Geometry: final body of the model. Coordinates: model frame, mm. Face numbers are marked on the shaded views. A direction names the side the tool comes from. Give positions to 0.01 mm unless a question says otherwise; leave off trailing zeros. Loops run counter-clockwise (first coordinate to the right, second up) from the corner with the lowest first, then second, coordinate; pieces in that order, holes last.
1. First-contact query: P1, Ø8, axis at y = 19.5, z = 1, coming from the +X side; P2, Ø6, axis at y = 23.5, z = 1, coming from the -X side. Flat tips, straight axial feed; report the tip coordinate or a pass-through.
2. Material intervals for line 1 along Y through (x, z) = (-0.75, 6.25); line 2 along Z through (x, y) = (-1.75, 23.5); line 3 along Y through (x, z) = (-2, -3), sorted ascending.
3. Section B-B, the plane y = 22. Output: boundary loops of the cut face in (x, z), then the cut area to 3 significant figures.
4. Section A-A, the plane y = 31. Output: boundary loops of the cut face in (x, z).
5. Access query for the marked faces 1 and 2. Directions: +Z, -Z, +X, -X, +Y, -Y. A direction counts if a zero-diameter tool reaches every point of the face in a straight line with its end or side. Return the directions, or none.
from build123d import *

# Parameters (mm, degrees)
SKETCH1_W           = 4
SKETCH1_H           = 30
BOSS_EXTRUDE1_DEPTH = 5.5
FILLET1_R           = 0.4
CHAMFER1_SIZE       = 0.4
SKETCH3_OUTSIDE_W   = 25.696
SKETCH3_OUTSIDE_H   = 27.708
SKETCH3_OUTSIDE_R   = 6.5
CUT_EXTRUDE1_DEPTH  = 1
CUT_EXTRUDE1_DRAFT  = -52


with BuildPart() as part:
    # Sketch1 → Revolve1 (revolve)
    with BuildSketch(Plane.XY, mode=Mode.PRIVATE) as revolve1_sk:
        with Locations((-2, 15)):
            Rectangle(SKETCH1_W, SKETCH1_H)
    revolve(revolve1_sk.sketch.rotate(Axis((0, 30, 0), (0, -1, 0)), 270), axis=Axis((0, 30, 0), (0, -1, 0)))

    # Sketch2 → Boss-Extrude1 (add)
    with BuildSketch(Plane(origin=(0, 30, 0), x_dir=(1, 0, 0), z_dir=(0, 1, 0))):
        Polygon((0, -7.505553499), (6.5, -3.75277675), (6.5, 3.75277675), (0, 7.505553499), (-6.5, 3.75277675), (-6.5, -3.75277675), align=None)
    extrude(amount=BOSS_EXTRUDE1_DEPTH)

    # Fillet1
    fillet1_edges = [part.edges().sort_by_distance(p)[0] for p in [
        (0, 30, -4),
    ]]
    fillet(fillet1_edges, radius=FILLET1_R)

    # Chamfer1
    chamfer1_edges = [part.edges().sort_by_distance(p)[0] for p in [
        (0, 0, -4),
    ]]
    chamfer(chamfer1_edges, length=CHAMFER1_SIZE)


with BuildPart() as cut_extrude1_tool:
    # Sketch3 outside → Cut-Extrude1 (with draft: the straight prism first)
    with BuildSketch(Plane(origin=(0, 35.5, 0), x_dir=(1, 0, 0), z_dir=(0, 1, 0))):
        Rectangle(SKETCH3_OUTSIDE_W, SKETCH3_OUTSIDE_H)
        Circle(SKETCH3_OUTSIDE_R, mode=Mode.SUBTRACT)
    extrude(amount=-CUT_EXTRUDE1_DEPTH)
    # Cut-Extrude1: the draft: its side faces are tilted about the plane it starts from
    cut_extrude1_sides = [cut_extrude1_tool.faces().sort_by_distance(p)[0] for p in [
        (0, 35, 13.854),
        (12.848, 35, 0),
        (0, 35, -13.854),
        (-12.848, 35, 0),
        (-6.5, 35, 0),
    ]]
    draft(cut_extrude1_sides, Plane(origin=(0, 35.5, 0), x_dir=(1, 0, 0), z_dir=(0, 1, 0)), CUT_EXTRUDE1_DRAFT)


with BuildPart() as part_1:
    add(part.part)

    # Cut-Extrude1: cut by cut_extrude1_tool
    add(cut_extrude1_tool.part, mode=Mode.SUBTRACT)


solid = part_1.part
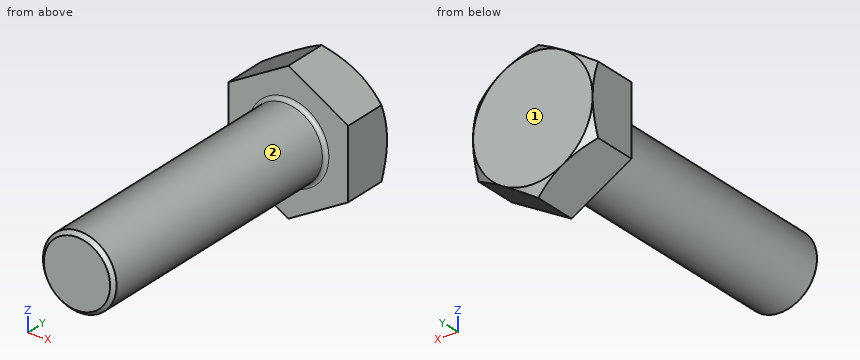
Answers below:
1. P1: stops at x = 4
1. P2: stops at x = -4
2. line 1: y = 30 to 35.5
2. line 2: z = -3.6 to 3.6
2. line 3: y = 0.01 to 35.5
3. outline: circle Ø8 at (0, 0)
3. area: 50.3 mm2
4. outline: (-6.5, -3.75) - (0, -7.51) - (6.5, -3.75) - (6.5, 3.75) - (0, 7.51) - (-6.5, 3.75) - close
5. face 1: +Z, -Z, +X, -X, +Y
5. face 2: -Y
